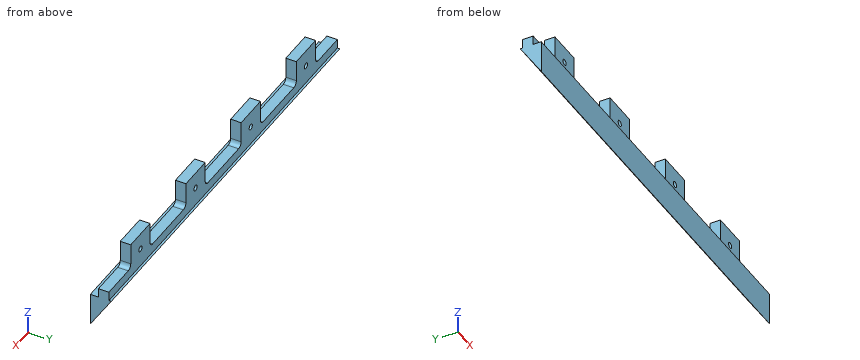
Autodesk Inventor part; units mm, degrees
ref_plane "YZ Plane" through (0, 0, 0) normal (1, 0, 0) x (0, 1, 0)
ref_plane "XZ Plane" through (0, 0, 0) normal (0, 1, 0) x (-1, 0, 0)
ref_plane "XY Plane" through (0, 0, 0) normal (0, 0, 1) x (1, 0, 0)
sketch "Sketch3" plane through (0, 0, 0) normal (1, 0, 0) x (0, 1, 0)
  line L0 (0, 0) -> (9, 0)
  line L1 (9, 0) -> (9, -14)
  line L2 (9, -14) -> (0, -14)
  line L3 (0, -14) -> (0, 0)
  line L4 (9, 0) -> (0, -14)
  line L5 (8, 0) -> (3.5, 0)
  line L6 (3.5, 0) -> (3.5, 15)
  line L7 (3.5, 15) -> (8, 15)
  line L8 (8, 15) -> (8, 0)
  line L9 (8.5, 0) -> (8, 0)
  line L10 (8, 0) -> (8, 4)
  point P0 (3.5, 0)
  dimension "d30" = 15
  dimension "d31" = 4.5
  dimension "d63" = 9
  dimension "d141" = 32.735
  dimension "d142" = 14
  dimension "d143" = 3.5
  dimension "d144" = 1
extrude "Extrusion2" add sketch "Sketch3" along normal blind 178 contours L0 L4 L3 | L6 L7 L8 L0
sketch "Sketch10" plane through (0, 3.5, -14) normal (0, -1, 0) x (1, 0, 0)
  line L0 (0, 14) -> (0, 26)
  line L1 (0, 26) -> (178, 26)
  line L2 (178, 14) -> (178, 26)
  line L3 (0, 14) -> (0, 18)
  line L4 (0, 18) -> (17, 18)
  line L5 (17, 18) -> (17, 26)
  line L6 (17, 26) -> (0, 26)
  line L7 (0, 26) -> (0, 18)
  line L8 (0, 18) -> (178, 18)
  line L9 (178, 26) -> (161, 26)
  line L10 (161, 26) -> (161, 18)
  line L11 (161, 18) -> (178, 18)
  line L12 (178, 18) -> (178, 26)
  line L13 (17, 26) -> (32, 26)
  line L14 (32, 26) -> (32, 18)
  line L15 (32, 18) -> (17, 18)
  line L16 (17, 18) -> (17, 26)
  line L17 (60, 26) -> (75, 26)
  line L18 (75, 26) -> (75, 18)
  line L19 (75, 18) -> (60, 18)
  line L20 (60, 18) -> (60, 26)
  line L21 (103, 26) -> (118, 26)
  line L22 (118, 26) -> (118, 18)
  line L23 (118, 18) -> (103, 18)
  line L24 (103, 18) -> (103, 26)
  line L25 (146, 26) -> (161, 26)
  line L26 (161, 26) -> (161, 18)
  line L27 (161, 18) -> (146, 18)
  line L28 (146, 18) -> (146, 26)
  line L29 (17, 26) -> (32, 18)
  line L30 (32, 26) -> (17, 18)
  line L31 (60, 26) -> (75, 18)
  line L32 (75, 26) -> (60, 18)
  line L33 (103, 26) -> (118, 18)
  line L34 (118, 26) -> (103, 18)
  line L35 (146, 26) -> (161, 18)
  line L36 (161, 26) -> (146, 18)
  line L37 (0, 14) -> (178, 14)
  line L38 (178, 26) -> (161, 26)
  line L39 (161, 26) -> (161, 33.1494)
  line L40 (161, 33.1494) -> (178, 33.1494)
  line L41 (178, 33.1494) -> (178, 26)
  line L42 (146, 26) -> (118, 26)
  line L43 (118, 26) -> (118, 37.5544)
  line L44 (118, 37.5544) -> (146, 37.5544)
  line L45 (146, 37.5544) -> (146, 26)
  line L46 (103, 26) -> (75, 26)
  line L47 (75, 26) -> (75, 36.0625)
  line L48 (75, 36.0625) -> (103, 36.0625)
  line L49 (103, 36.0625) -> (103, 26)
  line L50 (60, 26) -> (32, 26)
  line L51 (32, 26) -> (32, 34.4304)
  line L52 (32, 34.4304) -> (60, 34.4304)
  line L53 (60, 34.4304) -> (60, 26)
  line L54 (17, 26) -> (0, 26)
  line L55 (0, 26) -> (0, 37.0756)
  line L56 (0, 37.0756) -> (17, 37.0756)
  line L57 (17, 37.0756) -> (17, 26)
  point P0 (118, 26)
  point P1 (24.5, 22)
  point P2 (67.5, 22)
  point P3 (110.5, 22)
  point P4 (153.5, 22)
  dimension "d118" = 17
  dimension "d119" = 17
  dimension "d120" = 15
  dimension "d121" = 15
  dimension "d122" = 15
  dimension "d123" = 15
  dimension "d124" = 0
  dimension "d125" = 0
  dimension "d126" = 28
  dimension "d129" = 28
  dimension "d130" = 28
extrude "Extrusion5" cut sketch "Sketch10" against normal up to next contours L0 L1 L5 L4 | L55 L56 L57 L1 | L8 L10 L1 L2 | L14 L1 L20 L8 | L1 L39 L40 L41 | L51 L52 L53 L1 | L8 L22 L1 L28 | L18 L1 L24 L8 | L1 L43 L44 L45 | L47 L48 L49 L1
fillet "Fillet3" radius 2 8 edges at (161, 5.75, 4) (146, 5.75, 4) (118, 5.75, 4) (103, 5.75, 4) (75, 5.75, 4) (60, 5.75, 4) (32, 5.75, 4) (17, 5.75, 4)
sketch "Sketch11" plane through (0, 8, 0) normal (0, 1, 0) x (1, 0, 0)
  point P0 (0, 0)
  point P1 (24.5, -8)
  point P2 (67.5, -8)
  point P3 (110.5, -8)
  point P4 (153.5, -8)
hole "Hole5" at (24.5, 8, 8) at (67.5, 8, 8) at (110.5, 8, 8) at (153.5, 8, 8) direction (0, -1, 0) diameter 2.459 depth 8.8
equation "\"d126\" = d130"
equation "\"d129\" = d130"
properties part number "plog" material "Steel, Alloy"
For this review, take the finished solid that the model builds, in its own axes (mm). Round coordinates to 2 decimals unless told otherwise and drop trailing zeros. Write each loop counter-clockwise with the first axis right and the second up, starting at its lowest first coordinate (ties: lowest second). Pieces come first, ordered by that corner, then holes. Notation, with made-up numbers: M 40.25,54.5 L 51.25,54.5 A26 cw 51.25,87.5 Z; hole C 70,-15 d1. An arc over 180 degrees is marked long. Write item = value, one per line. Start each with the question number.
(1) We need section A-A (x = 96). Give the boundary of the cut face in (y, z), then the cut area to 3 significant figures.
(2) Clearance check with flat-ended pins moving along their axes: pin 1 Ø2 at (y, z) = (5, 10) entering from +X; pin 2 Ø2 at (x, y) = (4.5, 6) entering from +Z; pin 3 Ø2 at (y, z) = (5.5, 11) entering from -X. State where each tip first meets the part, or that it passes through.
(3) We need section B-B (y = 5.5). Give the number of separate pieces and of enclosed holes in the cut face, then the cut area to 3 significant figures.
(4) For line 1 along Z through (x, y) = (110.5, 6); line 2 along Z through (x, y) = (110.5, 6.9); line 3 along Y through (x, z) = (109, -0.75), list the stretches that pass through material, from the lowest coordinate up.
(5) We need section C-C (z = 1.5). Give the boundary of the cut face in (x, y).
Results found:
q1.outline = M 0,-14 L 9,0 L 8,0 L 8,4 L 3.5,4 L 3.5,0 L 0,0 Z
q1.area = 81.0 mm²
q2.pin_1 = 161
q2.pin_2 = 4
q2.pin_3 = 17
q3.separate_pieces = 1
q3.enclosed_holes = 4
q3.area = 2,330 mm²
q4.line_1 = -4.67 to 6.77, 9.23 to 15
q4.line_2 = -3.27 to 6.77, 9.23 to 15
q4.line_3 = 0 to 8.52
q5.outline = M 0,3.5 L 178,3.5 L 178,8 L 0,8 Z
